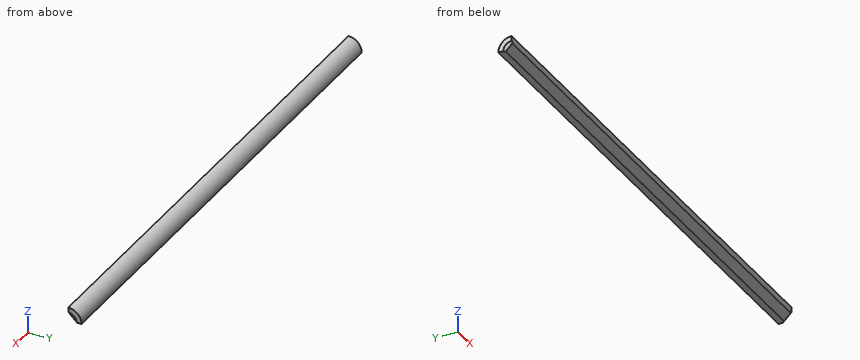
Autodesk Inventor part; units mm, degrees
ref_plane "YZ Plane" through (0, 0, 0) normal (1, 0, 0) x (0, 1, 0)
ref_plane "XZ Plane" through (0, 0, 0) normal (0, 1, 0) x (-1, 0, 0)
ref_plane "XY Plane" through (0, 0, 0) normal (0, 0, 1) x (1, 0, 0)
sketch "Sketch1" plane through (0, 0, 0) normal (1, 0, 0) x (0, 1, 0)
  line L0 (-6.35, 6.35) -> (6.35, 6.35)
  line L1 (6.35, 6.35) -> (6.35, -6.35)
  line L2 (6.35, -6.35) -> (-6.35, -6.35)
  line L3 (-6.35, -6.35) -> (-6.35, 6.35)
  line L4 (-6.35, 6.35) -> (6.35, -6.35) construction
  line L5 (6.35, 6.35) -> (-6.35, -6.35) construction
  point P0 (0, 0)
  dimension "d0" = 12.7
  dimension "d1" = 12.7
extrude "Extrusion1" add sketch "Sketch1" along normal mid plane 500
chamfer "Chamfer1" distance 6.35 angle 45 1 edges at (0, -6.35, -6.35)
fillet "Fillet1" radius 12.7 1 edges at (0, 6.35, 6.35)
sketch "Sketch2" plane through (250, 0, -6.35) normal (0, 0, -1) x (-1, 0, 0)
  line L0 (500, 0) -> (0, 0)
  line L1 (500, 6.35) -> (500, 0)
  line L2 (0, 6.35) -> (500, 6.35)
  line L3 (0, 0) -> (0, 6.35)
  circle A0 centre (500, 0) radius 1.5875
  line L4 (0, -6.35) -> (500, -6.35)
  line L5 (500, 0) -> (0, 0)
  line L6 (498.4125, 0) -> (498.4125, -6.35)
  line L7 (501.5875, 0) -> (501.5875, -6.35)
  line L8 (501.5875, -6.35) -> (498.4125, -6.35)
  point P0 (250, 0)
  dimension "d8" = 3.175
revolve "Revolution1" cut sketch "Sketch2" angle 360 about axis through (250, -6.35, -6.35) along (-1, 0, 0) contours L1 A0 L0 | L0 A0 L1 | A0 L7 L8 L4 L6
mirror "Mirror1" about plane through (0, 0, 0) normal (1, 0, 0) of "Revolution1"
equation "\"d0\" = facingThickness"
equation "\"d1\" = facingThickness"
equation "\"d2\" = depth"
equation "\"d4\" = 0.5 * facingThickness"
equation "\"d7\" = facingThickness"
equation "\"d8\" = 0.25 * facingThickness"
equation "\"depth\" = 500"
equation "\"facingThickness\" = 12.7"
equation "\"facingGasketThickness\" = 1.5875"
properties part number "sideMoulding" material "Wood (Cherry)"
CAD build for the part. Positions are in the model's coordinates, mm. Give positions to 0.01 mm unless a question says otherwise; leave off trailing zeros. Loops run counter-clockwise (first coordinate to the right, second up) from the corner with the lowest first, then second, coordinate; pieces in that order, holes last. Notation, with made-up numbers: M -1,3.5 L 3,3.5 A24 ccw 3,31.5 Z; hole C -4.5,40 d10. An arc over 180 degrees is marked long. Write each question's results on one line, items separated by ' | '.
Q1. Band-saw the part on C-C on y = 4.25. Write the cut outline in (x, z).
Geometry check:
outline: M -250,-6.35 L 250,-6.35 L 250,0.65 L -250,0.65 Z
Q2. Band-saw the part on B-B on z = 4. Write the cut outline in (x, y), and give its area (3 significant figures).
Geometry check:
outline: M -250,-6.35 L 250,-6.35 L 250,1.01 L -250,1.01 Z | area: 3,680 mm²
Q3. Probe probe 1 along Z at (x, y) = (142, 3.5); probe 2 along Z at (x, y) = (119, -4.25). List the from-to ranges inside material, lowest first.
Geometry check:
probe 1: z = -6.35 to 1.67 | probe 2: z = -2.1 to 6.18
Q4. Flat gauge pins, fed straight in: P1, Ø1.9, axis at y = -2.5, z = -3.5, coming from the -X side; P2, Ø3, axis at y = -2.5, z = -2.5, coming from the +X side. Where does each tip first touch, or does it go through?
Geometry check:
P1: stops at x = -248.41 | P2: stops at x = 248.53
